Could you check a few things on this model? Use its own coordinates, in mm. A direction names the side the tool comes from. Give positions to 0.01 mm unless a question says otherwise; leave off trailing zeros. Order: outer loops, then holes, each group sorted by start corner. A loop starts at its lowest first (then second) coordinate and runs counter-clockwise, first axis right, second up. Notation, with made-up numbers: M 41,5.25 L 85,5.25 A28 cw 85,42.25 Z; hole C -24.75,53.25 d6. An arc over 180 degrees is marked long. Answer in a Markdown table with one row per item. Add a question column.
```python
from build123d import *

# Parameters (mm, degrees)
SKETCH_R        = 11.3
SKETCH_R_2      = 1.6
SKETCH_R_3      = 3.2
PAD_DEPTH       = 15
SKETCH001_R     = 3.2
POCKET_DEPTH    = 4
SKETCH002_R     = 5.2
POCKET001_DEPTH = 5


with BuildPart() as part:
    # Sketch → Pad (new body)
    with BuildSketch(Plane.XY):
        Polygon((20, 30), (20, 51), (62.3, 51), (62.3, 30), (82.3, 30), (82.3, 0), (0, 0), (0, 30), align=None)
        with Locations((41.15, 29.85)):
            Circle(SKETCH_R, mode=Mode.SUBTRACT)
        with Locations((25.65, 45.35)):
            Circle(SKETCH_R_2, mode=Mode.SUBTRACT)
        with Locations((25.65, 14.35)):
            Circle(SKETCH_R_2, mode=Mode.SUBTRACT)
        with Locations((56.65, 45.35)):
            Circle(SKETCH_R_2, mode=Mode.SUBTRACT)
        with Locations((56.65, 14.35)):
            Circle(SKETCH_R_2, mode=Mode.SUBTRACT)
        with Locations((11.15, 10)):
            Circle(SKETCH_R_3, mode=Mode.SUBTRACT)
        with Locations((67.35, 10)):
            Circle(SKETCH_R_3, mode=Mode.SUBTRACT)
        with Locations((78.75, 10)):
            Circle(SKETCH_R_3, mode=Mode.SUBTRACT)
    extrude(amount=PAD_DEPTH)

    # Sketch001 (on Face18 of Pad) → Pocket (cut)
    with BuildSketch(Plane.XY.offset(15)):
        with Locations((25.65, 45.35)):
            Circle(SKETCH001_R)
        with Locations((56.65, 45.35)):
            Circle(SKETCH001_R)
        with Locations((56.65, 14.35)):
            Circle(SKETCH001_R)
        with Locations((25.65, 14.35)):
            Circle(SKETCH001_R)
    extrude(amount=-POCKET_DEPTH, mode=Mode.SUBTRACT)

    # Sketch002 (on Face4 of Pocket) → Pocket001 (cut)
    with BuildSketch(Plane(origin=(0, 0, 0), x_dir=(1, 0, 0), z_dir=(0, 0, -1))):
        with Locations((11.15, -10)):
            Circle(SKETCH002_R)
        with Locations((67.35, -10)):
            Circle(SKETCH002_R)
        with Locations((78.75, -10)):
            Circle(SKETCH002_R)
    extrude(amount=-POCKET001_DEPTH, mode=Mode.SUBTRACT)


solid = part.part
```
1. Suppose I cut it at A-A on x = 56.65. List the corners of the cut face in (y, z) for me.
2. Suppose I cut it at C-C on z = 6.5. Count the separate pieces of the cut face and the enclosed holes in it, plus the area to 3 significant figures.
3. Thinking about a two-plate mould opening in X: for faces 6 (the flat face through (82.3, 15, 7)), 7 (the cylindrical face through (28.702, 46.311, 13.028)), 8 (the flat face through (33, 20, 0)), 9 (the flat face through (75, 10, 5)), which applies, pulls with the +X half, pulls with the -X half, needs draft (parallel to the pull), parting line crosses it, or undercut?
4. Suppose I cut it at B-B on y = 45.35. List the corners of the cut face in (x, z) for me.
5. If I drill on line 1 along X through (y, z) = (10, 11); line 2 along Y through (x, z) = (11, 6.75); line 3 along X through (y, z) = (46, 14), over which ranges is the centre line in solid material (lowest first)? Write a range as [from, to].
6. Suppose I cut it at D-D on y = 10. List the corners of the cut face in (x, z) for me.
7. For faces 1 (the flat face through (0, 15, 7)), 2 (the cylindrical face through (73.553, 9.831, 2.465)), 3 (the flat face through (72, 30, 7)), 4 (the cylindrical face through (56.442, 15.936, 5.423)), 5 (the flat face through (55, 46, 11)), which set-ups out of +Z, -Z, +X, -X, +Y, -Y let a thin tool reach every point of the face, with its end or its side?
8. Will these pins go through, and if not, where does the flat tip stop? P1, Ø1.5, axis at x = 50, y = 23, coming from the -Z side; P2, Ø2.5, axis at x = 76.5, y = 9, coming from the -Z side; P3, Ø1, axis at y = 43, z = 5, coming from the +X side; P4, Ø3.5, axis at x = 25.65, y = 45.35, coming from the +Z side.
Findings below:
| question | item | result |
|---|---|---|
| 1 | outline | M 0,0 L 12.75,0 L 12.75,11 L 11.15,11 L 11.15,15 L 0,15 Z; M 15.95,0 L 43.75,0 L 43.75,11 L 42.15,11 L 42.15,15 L 17.55,15 L 17.55,11 L 15.95,11 Z; M 46.95,0 L 51,0 L 51,15 L 48.55,15 L 48.55,11 L 46.95,11 Z |
| 2 | separate pieces | 1 |
| 2 | enclosed holes | 8 |
| 2 | area | 2,830 mm2 |
| 3 | face 6 | pulls with the +X half |
| 3 | face 7 | undercut |
| 3 | face 8 | needs draft |
| 3 | face 9 | undercut |
| 4 | outline | M 20,0 L 24.05,0 L 24.05,11 L 22.45,11 L 22.45,15 L 20,15 Z; M 27.25,0 L 55.05,0 L 55.05,11 L 53.45,11 L 53.45,15 L 28.85,15 L 28.85,11 L 27.25,11 Z; M 58.25,0 L 62.3,0 L 62.3,15 L 59.85,15 L 59.85,11 L 58.25,11 Z |
| 5 | line 1 | [0, 7.95], [14.35, 64.15], [70.55, 75.55], [81.95, 82.3] |
| 5 | line 2 | [0, 6.8], [13.2, 30] |
| 5 | line 3 | [20, 22.52], [28.78, 53.52], [59.78, 62.3] |
| 6 | outline | M 0,0 L 5.95,0 L 5.95,5 L 7.95,5 L 7.95,15 L 0,15 Z; M 14.35,5 L 16.35,5 L 16.35,0 L 62.15,0 L 62.15,5 L 64.15,5 L 64.15,15 L 14.35,15 Z; M 70.55,5 L 72.55,5 L 72.55,0 L 73.55,0 L 73.55,5 L 75.55,5 L 75.55,15 L 70.55,15 Z; M 81.95,5 L 82.3,5 L 82.3,15 L 81.95,15 Z |
| 7 | face 1 | +Z, -Z, -X, +Y, -Y |
| 7 | face 2 | -Z |
| 7 | face 3 | +Z, -Z, +X, +Y |
| 7 | face 4 | +Z, -Z |
| 7 | face 5 | +Z |
| 8 | P1 | z = 0 |
| 8 | P2 | z = 5 |
| 8 | P3 | x = 62.3 |
| 8 | P4 | z = 11 |
